from build123d import *

# Parameters (mm, degrees)
SKETCH1_W                     = 582.097428288
SKETCH1_H                     = 518.453658302
BOSS_EXTRUDE1_DEPTH           = 414.782
BOSS_EXTRUDE1_TAPER           = 1
BOSS_EXTRUDE1_OTHER_WAY_DEPTH = 360.68
SKETCH2_R                     = 198.240238767
CUT_EXTRUDE1_DEPTH            = 868.899312363


with BuildPart() as part:
    # Sketch1 → Boss-Extrude1 (new body)
    with BuildSketch(Plane.XY):
        Rectangle(SKETCH1_W, SKETCH1_H)
    extrude(amount=BOSS_EXTRUDE1_DEPTH, taper=BOSS_EXTRUDE1_TAPER)

    # Sketch1 → Boss-Extrude1 other way (add)
    with BuildSketch(Plane.XY):
        Rectangle(SKETCH1_W, SKETCH1_H)
    extrude(amount=-BOSS_EXTRUDE1_OTHER_WAY_DEPTH)

    # Sketch2 → Cut-Extrude1 (cut, through all)
    with BuildSketch(Plane(origin=(0, 0, -360.68), x_dir=(-1, 0, 0), z_dir=(0, 0, -1))):
        with Locations((12.456248264, 0)):
            Circle(SKETCH2_R)
    extrude(amount=-CUT_EXTRUDE1_DEPTH, mode=Mode.SUBTRACT)


solid = part.part
For this review, take the finished solid that the model builds, in its own axes (mm). Give positions to 0.01 mm unless a question says otherwise; leave off trailing zeros. Order: outer loops, then holes, each group sorted by start corner. A loop starts at its lowest first (then second) coordinate and runs counter-clockwise, first axis right, second up. Notation, with made-up numbers: (83.25, -13) - (103.25, -13) arc R22 ccw to (103.25, 7) - close; hole circle Ø9 at (3, 59.25). An arc over 180 degrees is marked (long way). Answer as a JSON object with one key per item and string values. Group by question number.
Item 1: Take a section at B-B on x = 58. Give the boundary of the cut face in (y, z).
Item 2: Take a section at D-D on z = -255.5. Give the boundary of the cut face in (x, y), and give its area (3 significant figures).
Item 3: Draft analysis for pull direction Y (two halves, no side actions). For faces 1 (the flat face through (190, 4, -360.68)), 2 (the cylindrical face through (30.518, -193.526, 21.623)), 3 (the flat face through (-4, -259.227, -178)), 4 (the flat face through (-4, 259.227, -178)), state which applies: pulls with the +Y half, pulls with the -Y half, needs draft (parallel to the pull), parting line crosses it, or undercut.
Item 4: Clearance check with flat-ended pins moving along their axes: pin 1 Ø3 at (y, z) = (-15.5, 22) entering from +X; pin 2 Ø1.5 at (y, z) = (165.5, 101) entering from -X; pin 3 Ø1.5 at (y, z) = (-130, 188.5) entering from +X. State where each tip first meets the part, or that it passes through.
Item 5: Take a section at C-C on z = 50. Give the boundary of the cut face in (x, y), and give its area (3 significant figures).
Item 6: Take a section at A-A on y = 0. Give the boundary of the cut face in (x, z), and give its area (3 significant figures).
Item 7: Wall thickness on line 1 along X through (y, z) = (117, -308); line 2 along Y through (x, z) = (42.5, 201); line 3 along Y through (x, z) = (160.5, -235): over which ranges is each line inside the solid? List them lowest first.
Reported:
{
 "1": {"outline": "(-259.23, -360.68) - (-185.3, -360.68) - (-185.3, 414.78) - (-251.99, 414.78) - (-259.23, 0) - close; (185.3, -360.68) - (259.23, -360.68) - (259.23, 0) - (251.99, 414.78) - (185.3, 414.78) - close"},
 "2": {"outline": "(-291.05, -259.23) - (291.05, -259.23) - (291.05, 259.23) - (-291.05, 259.23) - close; hole circle Ø396.48 at (-12.46, 0)", "area": "178,000 mm^2"},
 "3": {"face 1": "needs draft", "face 2": "undercut", "face 3": "pulls with the -Y half", "face 4": "pulls with the +Y half"},
 "4": {"pin 1": "x = 290.69", "pin 2": "x = -289.3", "pin 3": "x = 287.77"},
 "5": {"outline": "(-290.18, -258.35) - (290.18, -258.35) - (290.18, 258.35) - (-290.18, 258.35) - close; hole circle Ø396.48 at (-12.46, 0)", "area": "176,000 mm^2"},
 "6": {"outline": "(-291.05, -360.68) - (-210.7, -360.68) - (-210.7, 414.78) - (-283.81, 414.78) - (-291.05, 0) - close; (185.78, -360.68) - (291.05, -360.68) - (291.05, 0) - (283.81, 414.78) - (185.78, 414.78) - close", "area": "141,000 mm^2"},
 "7": {"line 1": "-291.05 to -172.49, 147.58 to 291.05", "line 2": "-255.72 to -190.47, 190.47 to 255.72", "line 3": "-259.23 to -96.88, 96.88 to 259.23"}
}
